Could you check a few things on this model? Use its own coordinates, in mm. A direction names the side the tool comes from. Coordinates: 2 decimals unless noted, no trailing zeros. Loops run counter-clockwise (first coordinate to the right, second up) from the corner with the lowest first, then second, coordinate; pieces in that order, holes last.
Autodesk Inventor part; units mm, degrees
ref_plane "YZ Plane" through (0, 0, 0) normal (1, 0, 0) x (0, 1, 0)
ref_plane "XZ Plane" through (0, 0, 0) normal (0, 1, 0) x (-1, 0, 0)
ref_plane "XY Plane" through (0, 0, 0) normal (0, 0, 1) x (1, 0, 0)
sketch "Sketch1" plane through (0, 0, 0) normal (1, 0, 0) x (0, 1, 0)
  circle A0 centre (0, 0) radius 25.4
  line L0 (6.3913, -3.5936) -> (0.0835, -7.3319)
  line L1 (0.0835, -7.3319) -> (-6.3079, -3.7382)
  line L2 (-6.3079, -3.7382) -> (-6.3913, 3.5936)
  line L3 (-6.3913, 3.5936) -> (-0.0835, 7.3319)
  line L4 (-0.0835, 7.3319) -> (6.3079, 3.7382)
  line L5 (6.3079, 3.7382) -> (6.3913, -3.5936)
  dimension "d0" = 50.8
  dimension "d6" = 6.35
extrude "Extrusion1" add sketch "Sketch1" along normal blind 203.2 contours A0 | L0 L1 L2 L3 L4 L5
extrude "Extrusion2" cut sketch "Sketch1" along normal through all contours L0 L1 L2 L3 L4 L5
properties part number "Roller" material "Rubber"
1) Imagine slicing it at C-C on y = -4.5. List the corners of the cut face in (x, z) for me, plus the area to 3 significant figures.
2) Imagine slicing it at B-B on z = 0. List the corners of the cut face in (x, y) for me.
3) Will these pins go through, and if not, where does the flat tip stop? pin 1 (2 mm diameter, centred on x = 133, z = 13, fed in from -Y); pin 2 (8 mm diameter, centred on x = 21.5, z = -5, fed in from -Y); pin 3 (2 mm diameter, centred on x = 26.5, y = -15, fed in from -Z).
4) Imagine slicing it at A-A on x = 34.5. List the corners of the cut face in (y, z) for me.
5) If I drill on L1, parallel to Y at x = 75.5, z = -7; L2, parallel to Z at x = 150, y = 3.5; L3, parallel to Z at x = 131.5, y = 6, over which ranges is the centre line in solid material (lowest first)?
6) Imagine slicing it at D-D on y = 18. List the corners of the cut face in (x, z) for me.
7) For faces 1 (the flat face through (100.18, -3.07, -5.56)), 2 (the flat face through (203.2, 5, -5)), which set-ups out of +Z, -Z, +X, -X, +Y, -Y let a thin tool reach every point of the face, with its end or its side?
8) We'd pull the mould along Y, two halves only. Please class faces 3 (the flat face through (0, 5, -5)), 4 (the flat face through (100.178, -3.282, 5.437)), 5 (the cylindrical face through (100.178, -5.506, 24.796)): released by +Y, released by -Y, zero draft, split by the parting line, or undercut.
Solved:
1. outline: (0, -25) - (203.2, -25) - (203.2, -4.75) - (0, -4.75) - close; (0, 4.71) - (203.2, 4.71) - (203.2, 25) - (0, 25) - close
1. area: 8,240 mm2
2. outline: (0, -25.4) - (203.2, -25.4) - (203.2, -6.35) - (0, -6.35) - close; (0, 6.35) - (203.2, 6.35) - (203.2, 25.4) - (0, 25.4) - close
3. pin 1: stops at y = -22.39
3. pin 2: stops at y = -25.38
3. pin 3: stops at z = -21.19
4. outline: circle Ø50.8 at (0, 0); hole (-6.39, 3.59) - (-6.31, -3.74) - (0.08, -7.33) - (6.39, -3.59) - (6.31, 3.74) - (-0.08, 7.33) - close
5. L1: y = -24.42 to -0.51, 0.64 to 24.42
5. L2: z = -25.16 to -5.31, 5.32 to 25.16
5. L3: z = -24.68 to -3.83, 3.91 to 24.68
6. outline: (0, -17.92) - (203.2, -17.92) - (203.2, 17.92) - (0, 17.92) - close
7. face 1: +X, -X
7. face 2: +Z, -Z, +X, +Y, -Y
8. face 3: zero draft
8. face 4: undercut
8. face 5: split by the parting line
